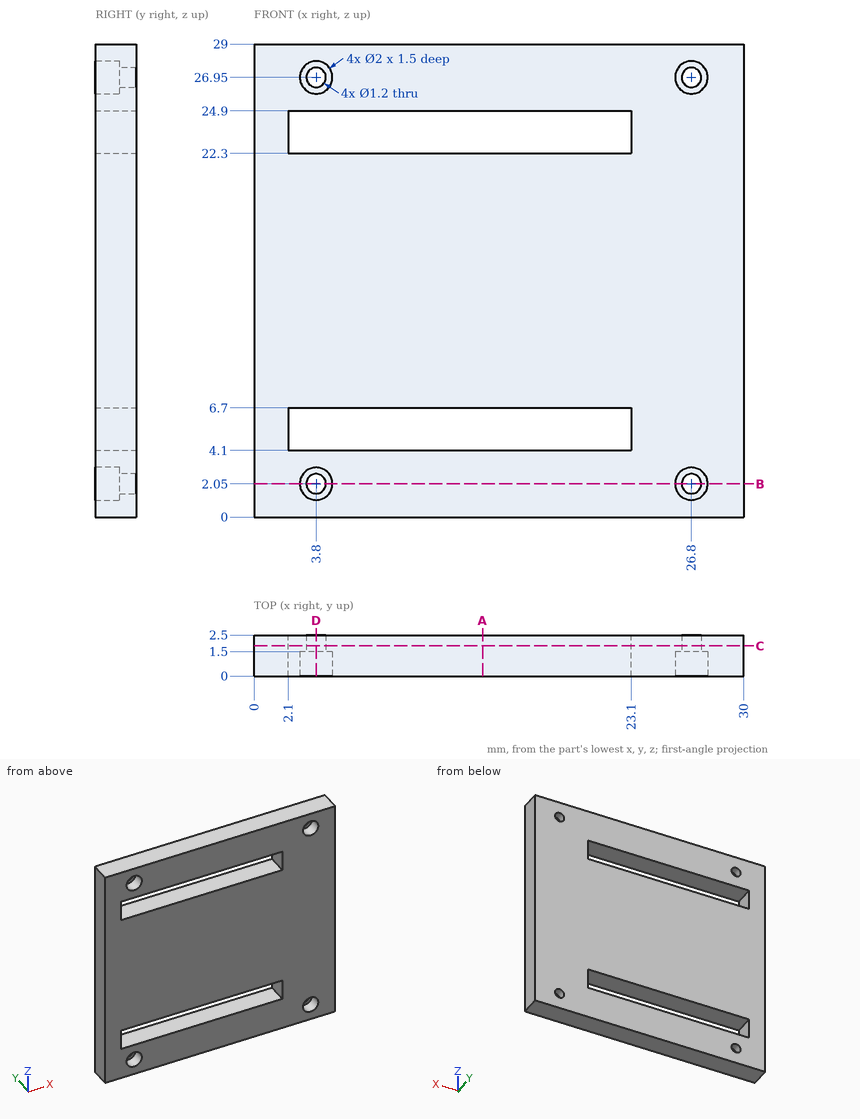
For this review, use the dimensioned drawing (mm, ordinates from the lowest corner) and the shaded views. Coordinates: 2 decimals unless noted, no trailing zeros. Loops run counter-clockwise (first coordinate to the right, second up) from the corner with the lowest first, then second, coordinate; pieces in that order, holes last. Notation, with made-up numbers: (38.25, -36.75) -> (91.25, -36.75) arc R16 ccw to (91.25, -11.75) -> close; hole circle Ø7 at (71, 2.25). An arc over 180 degrees is marked (long way). Use a Markdown table: item, result. Add a question column.
1. Add section C-C on y = 1.85. Write out the cut boundary in (x, z), plus the area to 3 significant figures.
2. Add section D-D on x = 3.8. Write out the cut boundary in (y, z), plus the area to 3 significant figures.
3. To check wall thickness, follow line 1 (Z direction, x = 10, y = 0.8); line 2 (X direction, y = 2.1, z = 2.05); line 3 (X direction, y = 0.9, z = 26.95). State the ranges of each line that lie inside material, in increasing order.
4. Add section A-A on x = 14. Write out the cut boundary in (y, z), plus the area to 3 significant figures.
5. Clearance check with a flat-ended pin moving along its axis: pin 1 Ø1.9 at (x, z) = (3.8, 2.05) entering from -Y. State where the tip first meets the part, or that it passes through.
6. Add section B-B on z = 2.05. Write out the cut boundary in (x, y).
Returned:
| question | item | result |
|---|---|---|
| 1 | outline | (0, 0) -> (30, 0) -> (30, 29) -> (0, 29) -> close; hole (2.1, 4.1) -> (23.1, 4.1) -> (23.1, 6.7) -> (2.1, 6.7) -> close; hole (2.1, 22.3) -> (23.1, 22.3) -> (23.1, 24.9) -> (2.1, 24.9) -> close; hole circle Ø1.2 at (3.8, 2.05); hole circle Ø1.2 at (3.8, 26.95); hole circle Ø1.2 at (26.8, 2.05); hole circle Ø1.2 at (26.8, 26.95) |
| 1 | area | 756 mm² |
| 2 | outline | (0, 0) -> (2.5, 0) -> (2.5, 1.45) -> (1.5, 1.45) -> (1.5, 1.05) -> (0, 1.05) -> close; (0, 3.05) -> (1.5, 3.05) -> (1.5, 2.65) -> (2.5, 2.65) -> (2.5, 4.1) -> (0, 4.1) -> close; (0, 6.7) -> (2.5, 6.7) -> (2.5, 22.3) -> (0, 22.3) -> close; (0, 24.9) -> (2.5, 24.9) -> (2.5, 26.35) -> (1.5, 26.35) -> (1.5, 25.95) -> (0, 25.95) -> close; (0, 27.95) -> (1.5, 27.95) -> (1.5, 27.55) -> (2.5, 27.55) -> (2.5, 29) -> (0, 29) -> close |
| 2 | area | 51.1 mm² |
| 3 | line 1 | z = 0 to 4.1, 6.7 to 22.3, 24.9 to 29 |
| 3 | line 2 | x = 0 to 3.2, 4.4 to 26.2, 27.4 to 30 |
| 3 | line 3 | x = 0 to 2.8, 4.8 to 25.8, 27.8 to 30 |
| 4 | outline | (0, 0) -> (2.5, 0) -> (2.5, 4.1) -> (0, 4.1) -> close; (0, 6.7) -> (2.5, 6.7) -> (2.5, 22.3) -> (0, 22.3) -> close; (0, 24.9) -> (2.5, 24.9) -> (2.5, 29) -> (0, 29) -> close |
| 4 | area | 59.5 mm² |
| 5 | pin 1 | stops at y = 1.5 |
| 6 | outline | (0, 0) -> (2.8, 0) -> (2.8, 1.5) -> (3.2, 1.5) -> (3.2, 2.5) -> (0, 2.5) -> close; (4.4, 1.5) -> (4.8, 1.5) -> (4.8, 0) -> (25.8, 0) -> (25.8, 1.5) -> (26.2, 1.5) -> (26.2, 2.5) -> (4.4, 2.5) -> close; (27.4, 1.5) -> (27.8, 1.5) -> (27.8, 0) -> (30, 0) -> (30, 2.5) -> (27.4, 2.5) -> close |
